from build123d import *

# Parameters (mm, degrees)
F0_R     = 12.7
F0_R_2   = 10.16
F1_DEPTH = 3.175
F2_DEPTH = 2.032
F0_R_3   = 3.3782
F3_DEPTH = 0.762
F4_R     = 8.4455
F5_DEPTH = 0.762
F7_D     = 6.7564


# Not quite as in the source:
# - the program builds the solid bodies; features that only make, move or delete a surface that nothing else refers to are left out


with BuildPart() as f1:
    # F0 (on Front) → F1 (new body)
    with BuildSketch(Plane.XZ):
        Circle(F0_R)
        Circle(F0_R_2, mode=Mode.SUBTRACT)
    extrude(amount=F1_DEPTH)

    # F0 (on Front) → F2 (join)
    with BuildSketch(Plane.XZ):
        Circle(F0_R_2)
        Polygon((1.4233928974, 5.3116902648), (5.3117551551, 1.4231507237), (3.8883622577, -3.8885395411), (-1.4233928974, -5.3116902648), (-5.3117551551, -1.4231507237), (-3.8883622577, 3.8885395411), align=None, mode=Mode.SUBTRACT)
    extrude(amount=F2_DEPTH)

    # F0 (on Front) → F3 (join)
    with BuildSketch(Plane.XZ):
        Polygon((3.8883622577, -3.8885395411), (5.3117551551, 1.4231507237), (1.4233928974, 5.3116902648), (-3.8883622577, 3.8885395411), (-5.3117551551, -1.4231507237), (-1.4233928974, -5.3116902648), align=None)
        Circle(F0_R_3, mode=Mode.SUBTRACT)
    extrude(amount=F3_DEPTH)

    # F4 (on face) → F5 (join)
    with BuildSketch(Plane.XZ):
        Circle(F4_R)
    extrude(amount=-F5_DEPTH)

    # F7 (through all)
    with Locations(Plane.XZ):
        with Locations((0, 0)):
            Hole(F7_D / 2)


solid = f1.part
The model under review builds one solid part; all positions refer to its coordinate system, in mm. A direction names the side the tool comes from. Round coordinates to 2 decimals unless told otherwise and drop trailing zeros. Loops run counter-clockwise (first coordinate to the right, second up) from the corner with the lowest first, then second, coordinate; pieces in that order, holes last. Notation, with made-up numbers: (26, 78.5) -> (67, 78.5) arc R17 cw to (67, 100.5) -> close; hole circle Ø11 at (-7.5, 13). An arc over 180 degrees is marked (long way). Answer as CSV lines item,"result".
1) To check wall thickness, follow line 1 along Z through (x, y) = (0, 0.55); line 2 along Z through (x, y) = (0, -2.75); line 3 along Y through (x, z) = (-0.5, 7). State the ranges of each line that lie inside material, in increasing order. Write a range as from..to.
Geometry results:
line 1,"z = -8.45..-3.38, 3.38..8.45"
line 2,"z = -12.7..-10.16, 10.16..12.7"
line 3,"y = -2.03..0.76"
2) Add section D-D on x = -6. Write out the cut boundary in (y, z) (3 decimals), plus the area to 3 significant figures.
Geometry results:
outline,"(-3.175, -11.193) -> (0, -11.193) -> (0, -5.944) -> (0.762, -5.944) -> (0.762, 5.944) -> (0, 5.944) -> (0, 11.193) -> (-3.175, 11.193) -> (-3.175, 8.199) -> (-2.032, 8.199) -> (-2.032, -8.199) -> (-3.175, -8.199) -> close"
area,"61.4 mm²"
3) Add section B-B on y = 0.35. Write out the cut boundary in (x, z).
Geometry results:
outline,"circle Ø16.89 at (0, 0); hole circle Ø6.76 at (0, 0)"
4) Draft analysis for pull direction X (two halves, no side actions). For faces 4 (the face through (-4.61, -1.39, 1.2)), 5 (the face through (-2.75, -1.57, -12.4)), 6 (the face through (4, 0.762, 0)), 7 (the face through (0, -0.762, 4)), state which applies: pulls with the +X half, pulls with the -X half, needs draft (parallel to the pull), parting line crosses it, or undercut.
Geometry results:
face 4,"undercut"
face 5,"parting line crosses it"
face 6,"needs draft"
face 7,"undercut"
5) For P1, Ø6, axis at x = 0, z = 0, coming from the +Y side; P2, Ø6, axis at x = -10, z = -9.5, coming from the +Y side; P3, Ø11.5, axis at x = 0, z = 2, coming from the -Y side; P4, Ø1, axis at x = 8, y = -1.5, coming from the +Z side, all flat-tipped, find the tip position at first contact; note any pin that passes through.
Geometry results:
P1,"passes through"
P2,"stops at y = 0"
P3,"stops at y = -2.03"
P4,"stops at z = 10.25"
6) Tool access review of faces 1 (the face through (-6, -3.175, 9)), 2 (the face through (-1.27, -1.39, 4.59)), 3 (the face through (2.6, 0, -8.3)): name each direction out of +Z, -Z, +X, -X, +Y, -Y from which nothing blocks a thin tool from reaching the whole face with its end or side.
Geometry results:
face 1,"+Z, -Z, +X, -X, -Y"
face 2,"-Y"
face 3,"+Y"
7) Add section A-A on x = 0. Write out the cut boundary in (y, z) (1 decimal), plus the area to 3 significant figures.
Geometry results:
outline,"(-3.2, -12.7) -> (0, -12.7) -> (0, -8.4) -> (0.8, -8.4) -> (0.8, -3.4) -> (-0.8, -3.4) -> (-0.8, -4.9) -> (-2, -4.9) -> (-2, -10.2) -> (-3.2, -10.2) -> close; (-3.2, 10.2) -> (-2, 10.2) -> (-2, 4.9) -> (-0.8, 4.9) -> (-0.8, 3.4) -> (0.8, 3.4) -> (0.8, 8.4) -> (0, 8.4) -> (0, 12.7) -> (-3.2, 12.7) -> close"
area,"47.5 mm²"
8) Add section C-C on z = 7. Write out the cut boundary in (x, y) (3 decimals).
Geometry results:
outline,"(-10.597, -3.175) -> (-7.364, -3.175) -> (-7.364, -2.032) -> (7.364, -2.032) -> (7.364, -3.175) -> (10.597, -3.175) -> (10.597, 0) -> (4.725, 0) -> (4.725, 0.762) -> (-4.725, 0.762) -> (-4.725, 0) -> (-10.597, 0) -> close"
